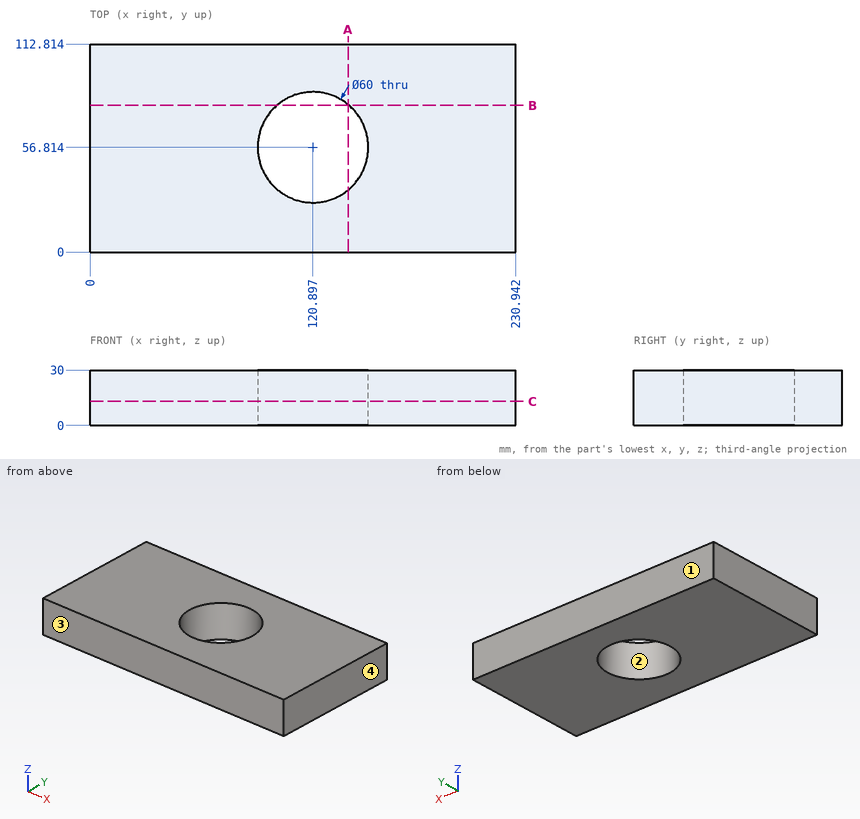
Part print with two shaded views. Sizes in mm from the minimum x, y, z corner. Round coordinates to 2 decimals unless told otherwise and drop trailing zeros. Loops run counter-clockwise (first coordinate to the right, second up) from the corner with the lowest first, then second, coordinate; pieces in that order, holes last.
1. Drill centre lines: line 1 along Y through (x, z) = (127, 7) (1 decimal); line 2 along Y through (x, z) = (110.5, 19.25) (1 decimal); line 3 along X through (y, z) = (31, 19.5) (1 decimal). Where is each one in solid material? Low to high.
Solutions:
line 1: y = 0 to 27.4, 86.2 to 112.8
line 2: y = 0 to 28.7, 85 to 112.8
line 3: x = 0 to 105.6, 136.2 to 230.9
2. Flat gauge pin, fed straight in: pin 1 (12 mm diameter, centred on x = 87.5, y = 99, fed in from -Z). Where does the tip first touch, or does it go through?
Solutions:
pin 1: stops at z = 0
3. Slice it at B-B (y = 79.5). Give the cut face in (x, z), and give its area (3 significant figures).
Solutions:
outline: (0, 0) - (101.27, 0) - (101.27, 30) - (0, 30) - close; (140.53, 0) - (230.94, 0) - (230.94, 30) - (140.53, 30) - close
area: 5,750 mm2
4. Slice it at A-A (x = 140). Give the cut face in (y, z) (1 decimal).
Solutions:
outline: (0, 0) - (33.7, 0) - (33.7, 30) - (0, 30) - close; (79.9, 0) - (112.8, 0) - (112.8, 30) - (79.9, 30) - close
5. Two-plate mould, pull along Y, no slides. Class the marked faces 1, 2, 3 and 4: pulls with the +Y half, pulls with the -Y half, needs draft (parallel to the pull), parting line crosses it, or undercut.
Solutions:
face 1: pulls with the +Y half
face 2: undercut
face 3: pulls with the -Y half
face 4: needs draft
6. Slice it at C-C (z = 13). Give the cut face in (x, y) (1 decimal).
Solutions:
outline: (0, 0) - (230.9, 0) - (230.9, 112.8) - (0, 112.8) - close; hole circle Ø60 at (120.9, 56.8)
